from build123d import *

# Parameters (mm, degrees)
F0_W     = 50
F0_H     = 50
F1_DEPTH = 50
F2_W     = 7.5
F2_H     = 7.5
F3_DEPTH = 50
F4_W     = 50
F4_H     = 50
F5_DEPTH = 50


with BuildPart() as f1:
    # F0 (on Top) → F1 (new body)
    with BuildSketch(Plane.XY):
        Rectangle(F0_W, F0_H)
    extrude(amount=F1_DEPTH)

    # F2 (on face) → F3 (join)
    with BuildSketch(Plane.XY.offset(50)):
        Polygon((15, 25), (-25, 25), (-25, -15), (-7.5, -15), (-7.5, 7.5), (15, 7.5), align=None)
        with Locations((11.25, -11.25)):
            Rectangle(F2_W, F2_H)
    extrude(amount=F3_DEPTH)

    # F4 (on face) → F5 (join)
    with BuildSketch(Plane.XY.offset(100)):
        Rectangle(F4_W, F4_H)
    extrude(amount=F5_DEPTH)


solid = f1.part
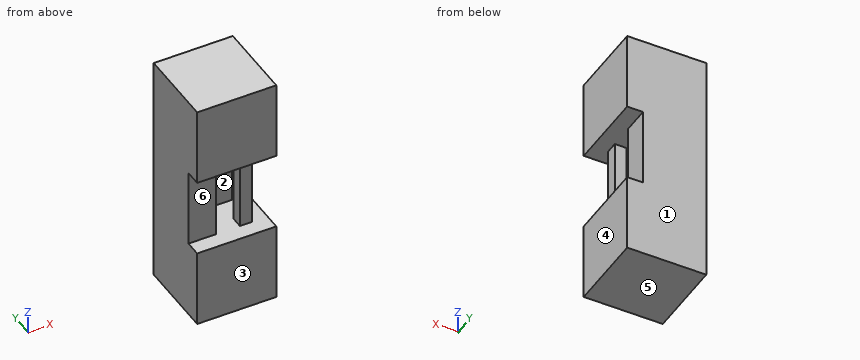
Verification items for the finished model (mm, model axes). Face numbers are marked on the shaded views. A direction names the side the tool comes from. Round coordinates to 2 decimals unless told otherwise and drop trailing zeros. Loops run counter-clockwise (first coordinate to the right, second up) from the corner with the lowest first, then second, coordinate; pieces in that order, holes last. Notation, with made-up numbers: (68.5, -15.5) - (127.5, -15.5) arc R4 ccw to (127.5, -8.5) - close; hole circle Ø7 at (86, 82.5). An arc over 180 degrees is marked (long way). Use a Markdown table: item, result. Add a question column.
1. Section check D-D, the plane y = 5.5. Record the boundary of the cut face in (x, z), plus the area to 4 significant figures.
2. Release check for a two-part mould opening along Y. For the marked faces 1, 2, 3 and 4 record: released by +Y, released by -Y, zero draft, split by the parting line, or undercut.
3. Section check C-C, the plane x = 10.5. Record the boundary of the cut face in (y, z), plus the area to 3 significant figures.
4. Access from +Z, -Z, +X, -X, +Y, -Y to the whole of each face (thin tool, end or side, straight path). Record for the marked faces 5 and 6.
5. Thickness scan on probe 1 along Z at (x, y) = (-2, -19); probe 2 along X at (y, z) = (-10.5, 93); probe 3 along Y at (x, z) = (9.5, 63.5). Record the ranges inside material, lowest first. Write a range as [from, to].
6. Section check B-B, the plane x = 17. Record the boundary of the cut face in (y, z), plus the area to 3 significant figures.
7. Section check A-A, the plane z = 57.5. Record the boundary of the cut face in (x, y), plus the area to 3 significant figures.
8. Gauge pin test, flat ends, axial feed: pin 1 (19 mm diameter, centred on x = -17, z = 80.5, fed in from -Y); pin 2 (7 mm diameter, centred on y = -3.5, z = 69, fed in from +X); pin 3 (19 mm diameter, centred on y = 19, z = 75.5, fed in from +X). Record the tip position at first contact, or that the pin passes through.
Checks:
| question | item | result |
|---|---|---|
| 1 | outline | (-25, 0) - (25, 0) - (25, 50) - (-7.5, 50) - (-7.5, 100) - (25, 100) - (25, 150) - (-25, 150) - close |
| 1 | area | 5,875 mm^2 |
| 2 | face 1 | released by +Y |
| 2 | face 2 | undercut |
| 2 | face 3 | released by -Y |
| 2 | face 4 | zero draft |
| 3 | outline | (-25, 0) - (25, 0) - (25, 150) - (-25, 150) - (-25, 100) - (-15, 100) - (-15, 50) - (-25, 50) - close; hole (-7.5, 50) - (7.5, 50) - (7.5, 100) - (-7.5, 100) - close |
| 3 | area | 6,250 mm^2 |
| 4 | face 5 | -Z, +X, -X, +Y, -Y |
| 4 | face 6 | +X, -X, -Y |
| 5 | probe 1 | z = [0, 50], [100, 150] |
| 5 | probe 2 | x = [-25, -7.5], [7.5, 15] |
| 5 | probe 3 | y = [-15, -7.5], [7.5, 25] |
| 6 | outline | (-25, 0) - (25, 0) - (25, 50) - (-25, 50) - close; (-25, 100) - (25, 100) - (25, 150) - (-25, 150) - close |
| 6 | area | 5,000 mm^2 |
| 7 | outline | (-25, -15) - (-7.5, -15) - (-7.5, 7.5) - (15, 7.5) - (15, 25) - (-25, 25) - close; (7.5, -15) - (15, -15) - (15, -7.5) - (7.5, -7.5) - close |
| 7 | area | 1,150 mm^2 |
| 8 | pin 1 | stops at y = -15 |
| 8 | pin 2 | stops at x = -7.5 |
| 8 | pin 3 | stops at x = 15 |
